Geometry check sheet. Reference: the model listing, model coordinates, mm. A direction names the side the tool comes from. Give positions to 0.01 mm unless a question says otherwise; leave off trailing zeros. Order: outer loops, then holes, each group sorted by start corner. A loop starts at its lowest first (then second) coordinate and runs counter-clockwise, first axis right, second up.
Autodesk Inventor part; units mm, degrees
ref_plane "ip_st_1_1_XY" through (2.5, 4.25, 0) normal (1, 0, 0) x (0, 0, -1)
ref_plane "ip_st_1_1_YZ" through (2.5, 4.25, 0) normal (0, 0, -1) x (0, 1, 0)
ref_plane "ip_st_1_1_ZX" through (2.5, 4.25, 0) normal (0, 1, 0) x (1, 0, 0)
sketch "Sketch_2" plane through (0, 0, 0) normal (0, 0, 1) x (1, 0, 0)
  line L0 (5, 0) -> (0, 0)
  arc A0 (0, 2.2) -> (0.2, 2) centre (0.2, 2.2) ccw
  line L1 (0.2, 2) -> (4.8, 2)
  arc A1 (4.8, 2) -> (5, 2.2) centre (4.8, 2.2) ccw
  line L2 (5, 2.2) -> (5, 3)
  line L3 (5, 3) -> (4.6875, 3)
  line L4 (4.6875, 3) -> (4.6875, 3.475)
  line L5 (4.6875, 3.475) -> (3.6054, 3.475)
  arc A2 (1.3946, 3.475) -> (3.6054, 3.475) centre (2.5, 4.25) ccw
  line L6 (1.3946, 3.475) -> (0.3125, 3.475)
  line L7 (0.3125, 3.475) -> (0.3125, 3)
  line L8 (0.3125, 3) -> (0, 3)
  line L9 (0, 3) -> (0, 2.2)
revolve "Revolution1" add sketch "Sketch_2" angle 360 about axis through (5, 0, 0) along (1, 0, 0)
ref_plane "ip_st_1_1_XY" through (2.5, 4.25, 0) normal (1, 0, 0) x (0, 0, -1)
ref_plane "ip_st_1_1_YZ" through (2.5, 4.25, 0) normal (0, 0, -1) x (0, 1, 0)
ref_plane "ip_st_1_1_ZX" through (2.5, 4.25, 0) normal (0, 1, 0) x (1, 0, 0)
ref_plane "ip_st_1_2_XY" through (2.5, 2.6498, 3.3228) normal (1, 0, 0) x (0, 0, -1)
ref_plane "ip_st_1_2_YZ" through (2.5, 2.6498, 3.3228) normal (0, 0, -1) x (0, 1, 0)
ref_plane "ip_st_1_2_ZX" through (2.5, 2.6498, 3.3228) normal (0, 1, 0) x (1, 0, 0)
ref_plane "ip_st_1_3_XY" through (2.5, -0.9457, 4.1434) normal (1, 0, 0) x (0, 0, -1)
ref_plane "ip_st_1_3_YZ" through (2.5, -0.9457, 4.1434) normal (0, 0, -1) x (0, 1, 0)
ref_plane "ip_st_1_3_ZX" through (2.5, -0.9457, 4.1434) normal (0, 1, 0) x (1, 0, 0)
ref_plane "ip_st_1_4_XY" through (2.5, -3.8291, 1.844) normal (1, 0, 0) x (0, 0, -1)
ref_plane "ip_st_1_4_YZ" through (2.5, -3.8291, 1.844) normal (0, 0, -1) x (0, 1, 0)
ref_plane "ip_st_1_4_ZX" through (2.5, -3.8291, 1.844) normal (0, 1, 0) x (1, 0, 0)
ref_plane "ip_st_1_5_XY" through (2.5, -3.8291, -1.844) normal (1, 0, 0) x (0, 0, -1)
ref_plane "ip_st_1_5_YZ" through (2.5, -3.8291, -1.844) normal (0, 0, -1) x (0, 1, 0)
ref_plane "ip_st_1_5_ZX" through (2.5, -3.8291, -1.844) normal (0, 1, 0) x (1, 0, 0)
ref_plane "ip_st_1_6_XY" through (2.5, -0.9457, -4.1434) normal (1, 0, 0) x (0, 0, -1)
ref_plane "ip_st_1_6_YZ" through (2.5, -0.9457, -4.1434) normal (0, 0, -1) x (0, 1, 0)
ref_plane "ip_st_1_6_ZX" through (2.5, -0.9457, -4.1434) normal (0, 1, 0) x (1, 0, 0)
ref_plane "ip_st_1_7_XY" through (2.5, 2.6498, -3.3228) normal (1, 0, 0) x (0, 0, -1)
ref_plane "ip_st_1_7_YZ" through (2.5, 2.6498, -3.3228) normal (0, 0, -1) x (0, 1, 0)
ref_plane "ip_st_1_7_ZX" through (2.5, 2.6498, -3.3228) normal (0, 1, 0) x (1, 0, 0)
ref_plane "ip_st_1a_XY" through (0, 0, 0) normal (1, 0, 0) x (0, 0, -1)
ref_plane "ip_st_1a_YZ" through (0, 0, 0) normal (0, 0, -1) x (0, 1, 0)
ref_plane "ip_st_1a_ZX" through (0, 0, 0) normal (0, 1, 0) x (1, 0, 0)
ref_plane "ip_st_2a_XY" through (0.3125, 0, 0) normal (1, 0, 0) x (0, 0, -1)
ref_plane "ip_st_2a_YZ" through (0.3125, 0, 0) normal (0, 0, -1) x (0, 1, 0)
ref_plane "ip_st_2a_ZX" through (0.3125, 0, 0) normal (0, 1, 0) x (1, 0, 0)
properties part number "F624ZZ Inner Ring"
Item 1: Set-up check for faces 4 (the cylindrical face through (0.846, -0.753, 3.392)), 5 (the flat face through (0.312, -3, -1)), 6 (the flat face through (4.688, -3, -1)): record each of +Z, -Z, +X, -X, +Y, -Y from which the full face is reachable in a straight line by a thin tool's end or side.
Reported:
face 4: +X, -X
face 5: -X
face 6: +X
Item 2: Draft check along Y on faces 1 (the flat face through (0, -2, 2)), 2 (the cylindrical face through (3, 0, -2)), 3 (the cylindrical face through (0.154, -2.997, -0.132)). Enter one of: released by +Y, released by -Y, zero draft, split by the parting line, or undercut.
Reported:
face 1: zero draft
face 2: undercut
face 3: split by the parting line
Item 3: Sectioned sample at D-D (x = 2.4). Enter the section's corners in (y, z).
Reported:
outline: circle Ø5.81 at (0, 0); hole circle Ø4 at (0, 0)
Item 4: Sectioned sample at C-C (x = 3.8). Enter the section's corners in (y, z) (3 decimals), and give its area (3 significant figures).
Reported:
outline: circle Ø6.95 at (0, 0); hole circle Ø4 at (0, 0)
area: 25.4 mm2
Item 5: Gauge pin test, flat ends, axial feed: pin 1 (1.5 mm diameter, centred on y = 0.5, z = 1.5, fed in from -X); pin 2 (1.5 mm diameter, centred on x = 4.5, z = 1, fed in from -Y); pin 3 (2 mm diameter, centred on x = 1, y = 2.5, fed in from +Z). Record the tip position at first contact, or that the pin passes through.
Reported:
pin 1: stops at x = 0
pin 2: stops at y = -3.47
pin 3: stops at z = 3.13
Item 6: Scan lines: L1, parallel to Z at x = 3.7, y = 0 (3 decimals); L2, parallel to Y at x = 3, z = 1.5; L3, parallel to Z at x = 2.2, y = 0. Record each from-to range of solid material in increasing order.
Reported:
L1: z = -3.475 to -2, 2 to 3.475
L2: y = -2.59 to -1.32, 1.32 to 2.59
L3: z = -2.93 to -2, 2 to 2.93
